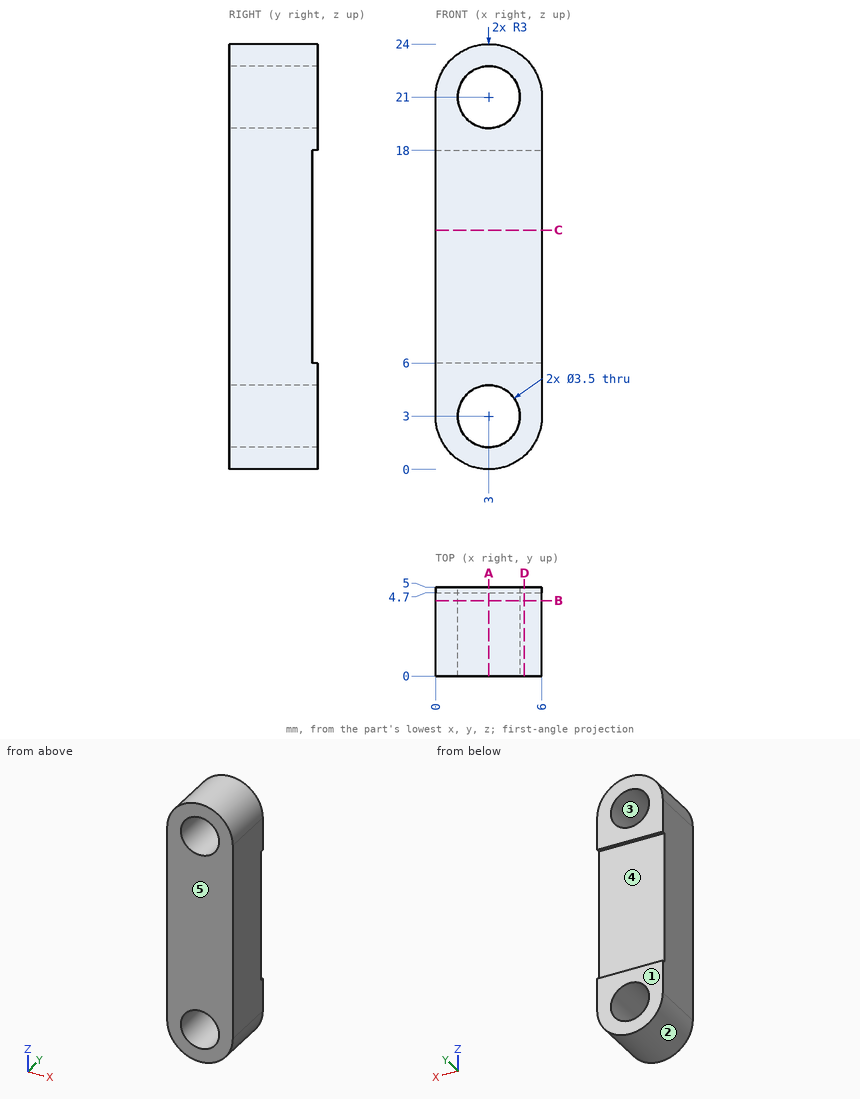
Geometry check sheet. Reference: drawing and pictorial views, mm from the part's lowest x, y, z. A direction names the side the tool comes from. Round coordinates to 2 decimals unless told otherwise and drop trailing zeros. Loops run counter-clockwise (first coordinate to the right, second up) from the corner with the lowest first, then second, coordinate; pieces in that order, holes last. Notation, with made-up numbers: M 83.5,9.5 L 135.5,9.5 A23 ccw 135.5,28.5 Z; hole C -37,-17 d6. An arc over 180 degrees is marked long. Return JSON: item names as keys, results as strings. Group by question number.
(1) Scan lines: line 1 along Z through (x, y) = (3, 1.95); line 2 along X through (y, z) = (3.05, 3); line 3 along Y through (x, z) = (0.55, 13.5). Record each from-to range of solid material in increasing order. Write a range as [from, to].
(2) Section check D-D, the plane x = 5. Enter the section's corners in (y, z).
(3) Set-up check for the marked faces 4 and 5: record each of +Z, -Z, +X, -X, +Y, -Y from which the full face is reachable in a straight line by a thin tool's end or side.
(4) Section check C-C, the plane z = 13.5. Enter the section's corners in (x, y).
(5) Section check A-A, the plane x = 3. Enter the section's corners in (y, z), and give its area (3 significant figures).
(6) Mould release check, pull along Z, two halves, no side actions. Record for the marked faces 1, 2 and 3: pulls with the +Z half, pulls with the -Z half, needs draft (parallel to the pull), parting line crosses it, or undercut.
(7) Go/stop test with flat-tipped pins: pin 1 (3 mm diameter, centred on x = 3, z = 3, fed in from -Y); pin 2 (3 mm diameter, centred on x = 3.5, z = 11.5, fed in from +Y). Record where each tip stops, or that it passes through.
(8) Section check B-B, the plane y = 4.25. Enter the section's corners in (x, z).
Data:
{
 "1": {"line 1": "[0, 1.25], [4.75, 19.25], [22.75, 24]", "line 2": "[0, 1.25], [4.75, 6]", "line 3": "[0, 4.7]"},
 "2": {"outline": "M 0,0.76 L 5,0.76 L 5,6 L 4.7,6 L 4.7,18 L 5,18 L 5,23.24 L 0,23.24 Z"},
 "3": {"face 4": "+X, -X, +Y", "face 5": "+Z, -Z, +X, -X, -Y"},
 "4": {"outline": "M 0,0 L 6,0 L 6,4.7 L 0,4.7 Z"},
 "5": {"outline": "M 0,0 L 5,0 L 5,1.25 L 0,1.25 Z; M 0,4.75 L 5,4.75 L 5,6 L 4.7,6 L 4.7,18 L 5,18 L 5,19.25 L 0,19.25 Z; M 0,22.75 L 5,22.75 L 5,24 L 0,24 Z", "area": "81.4 mm²"},
 "6": {"face 1": "needs draft", "face 2": "pulls with the -Z half", "face 3": "undercut"},
 "7": {"pin 1": "through", "pin 2": "y = 4.7"},
 "8": {"outline": "M 0,3 A3 ccw 6,3 L 6,21 A3 ccw 0,21 Z; hole C 3,3 d3.5; hole C 3,21 d3.5"}
}
